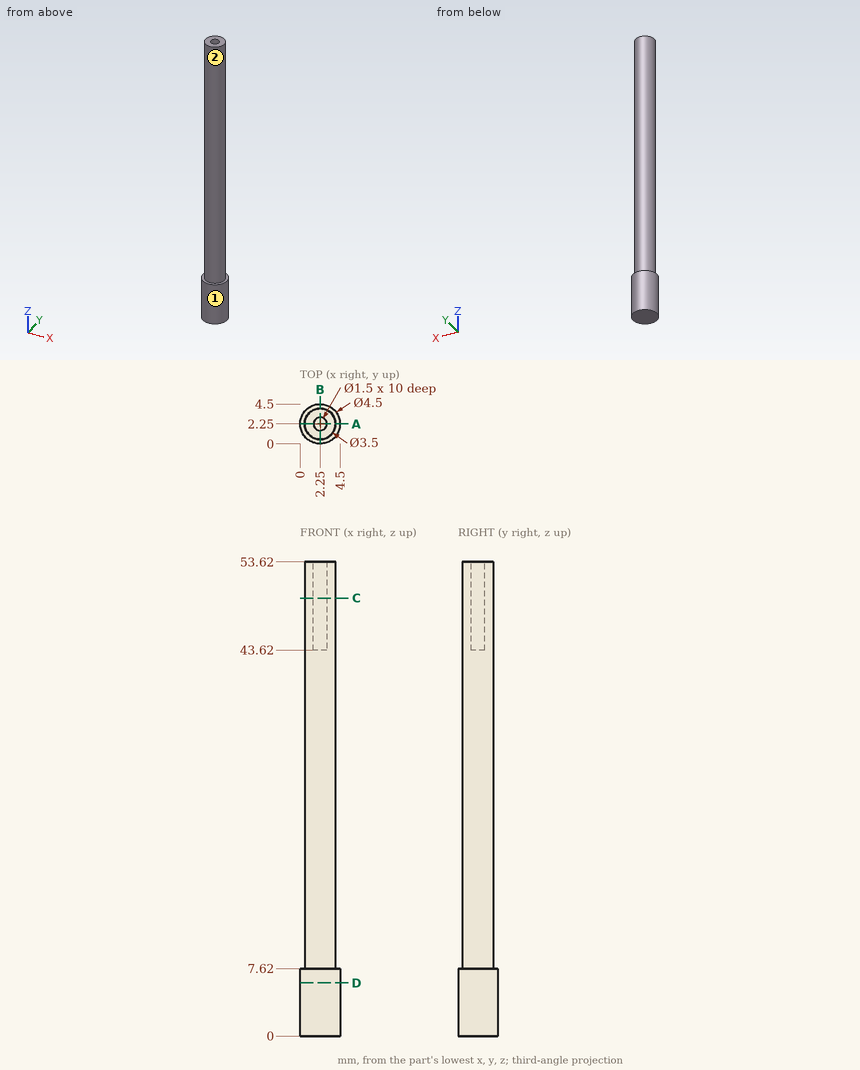
Design review of the part shown in the three views and the two pictorial views. Dimensions are in mm from the part's minimum x, y and z. A direction names the side the tool comes from. Round coordinates to 2 decimals unless told otherwise and drop trailing zeros. Loops run counter-clockwise (first coordinate to the right, second up) from the corner with the lowest first, then second, coordinate; pieces in that order, holes last. Notation, with made-up numbers: (20, 29) -> (26, 29) arc R15 ccw to (26, 58) -> close; hole circle Ø11 at (-24, 30). An arc over 180 degrees is marked (long way). Answer as a JSON object with one key per item and string values. Group by question number.
1) We need section A-A on y = 2.25. Write out the cut boundary in (x, z).
2) For the marked faces 1 and 2, list the 3-axis set-ups (+Z, -Z, +X, -X, +Y, -Y) from which the entire face can be reached by the end or side of a thin tool; tool diameter is ignored.
3) We need section D-D on z = 6. Write out the cut boundary in (x, y).
4) We need section C-C on z = 49.5. Write out the cut boundary in (x, y).
5) For line 1 (Y direction, x = 2.25, z = 51); line 2 (Z direction, x = 2.3, y = 2.7); line 3 (Z direction, x = 3.1, y = 0.6), list the stretches that pass through material, from the lowest coordinate up. Write a range as [from, to].
Result set:
{
 "1": {"outline": "(0, 0) -> (4.5, 0) -> (4.5, 7.62) -> (4, 7.62) -> (4, 53.62) -> (3, 53.62) -> (3, 43.62) -> (1.5, 43.62) -> (1.5, 53.62) -> (0.5, 53.62) -> (0.5, 7.62) -> (0, 7.62) -> close"},
 "2": {"face 1": "+Z, -Z", "face 2": "+Z"},
 "3": {"outline": "circle Ø4.5 at (2.25, 2.25)"},
 "4": {"outline": "circle Ø3.5 at (2.25, 2.25); hole circle Ø1.5 at (2.25, 2.25)"},
 "5": {"line 1": "[0.5, 1.5], [3, 4]", "line 2": "[0, 43.62]", "line 3": "[0, 7.62]"}
}
